Autodesk Fusion 360 part; units mm, degrees
sketch "Sketch1" plane through (0, 0, 0) normal (0, 0, 1) x (1, 0, 0)
  line L0 (9, 9) -> (-9, 9)
  line L1 (-9, 9) -> (-9, -9)
  line L2 (-9, -9) -> (9, -9)
  line L3 (9, -9) -> (9, 9)
  line L4 (9, 9) -> (-9, -9) construction
  line L5 (-9, 9) -> (9, -9) construction
  dimension "d1" = 18
  dimension "d2" = 18
extrude "Extrude1" add sketch "Sketch1" along normal blind 35

Autodesk Fusion 360 part; units mm, degrees
sketch "Sketch1" plane through (0, 0, 0) normal (0, 0, 1) x (1, 0, 0)
  line L0 (-10, -10) -> (10, -10)
  line L1 (10, -10) -> (10, 10)
  line L2 (10, 10) -> (-10, 10)
  line L3 (-10, 10) -> (-10, -10)
  line L4 (-10, -10) -> (10, 10) construction
  line L5 (10, -10) -> (-10, 10) construction
  dimension "d1" = 20
  dimension "d2" = 20
extrude "Extrude1" add sketch "Sketch1" along normal blind 65
sketch "Sketch2" plane through (0, 0, 0) normal (0, 0, -1) x (1, 0, 0)
  line L0 (-10, 10) -> (-10, -10)
  line L1 (-10, -10) -> (10, -10)
  line L2 (10, -10) -> (10, 10)
  line L3 (10, 10) -> (-10, 10)
  line L4 (10, 10) -> (10, -10)
  line L5 (10, -10) -> (10, 10)
  line L6 (10, 10) -> (30, 10) construction
  line L7 (30, 10) -> (30, -10) construction
  line L8 (30, -10) -> (10, -10) construction
  arc A0 (20, -10) -> (20, 10) centre (20, 0) ccw
  line L9 (20, -10) -> (10, -10) construction
  line L10 (10, -10) -> (10, 10) construction
  line L11 (20, -10) -> (10, -10)
  line L12 (20, 10) -> (10, 10)
  point P0 (10, -10)
  point P1 (10, 10)
  dimension "d5" = 20
extrude "Extrude2" add sketch "Sketch2" against normal blind 10 contours L2 L4 L5 A0 L11 L12
sketch "Sketch4" plane through (0, 0, 10) normal (0, 0, 1) x (-1, 0, 0)
  arc A0 (-20, 10) -> (-20, -10) centre (-20, 0) ccw
  line L0 (-20, -10) -> (-10, -10)
  line L1 (-10, -10) -> (-10, 10)
  line L2 (-10, 10) -> (-20, 10)
  line L3 (-20, 10) -> (-20, -10) construction
  point P0 (-20, 10)
  point P1 (-20, -10)
hole "Hole1" at (20, 0, 10) direction (0, 0, -1) diameter 6.5 depth 10 tip angle 180 counterbore diameter 11 counterbore depth 4
sketch "Sketch5" plane through (0, 0, 0) normal (0, 0, -1) x (1, 0, 0)
  circle A0 centre (20, 0) radius 3.25
  line L0 (-10, 10) -> (-10, -10)
  line L1 (-10, -10) -> (20, -10)
  arc A1 (20, -10) -> (20, 10) centre (20, 0) ccw
  line L2 (20, 10) -> (-10, 10)
  line L3 (6, 3.8) -> (-6, 3.8)
  line L4 (-6, 3.8) -> (-6, -3.8)
  line L5 (-6, -3.8) -> (6, -3.8)
  line L6 (6, -3.8) -> (6, 3.8)
  line L7 (6, 3.8) -> (-6, -3.8) construction
  line L8 (-6, 3.8) -> (6, -3.8) construction
  dimension "d13" = 12
  dimension "d14" = 7.6
extrude "Extrude3" add sketch "Sketch5" along normal blind 2 contours L3 L4 L5 L6
fillet "Fillet1" radius 1.5 11 edges at (-10, 10, 32.5) (-10, -10, 32.5) (10, -10, 37.5) (15, -10, 10) (30, 0, 10) (15, 10, 10) (10, 10, 37.5) (6, 3.8, -1) (6, -3.8, -1) (-6, -3.8, -1) (-6, 3.8, -1)
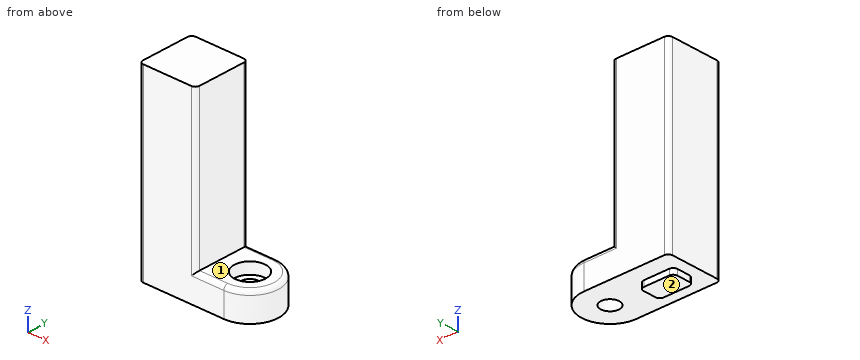
Check sheet for the modelled part. Datum: model origin and axes. Units: mm. Face numbers are marked on the shaded views. A direction names the side the tool comes from. Give positions to 0.01 mm unless a question says otherwise; leave off trailing zeros. Order: outer loops, then holes, each group sorted by start corner. A loop starts at its lowest first (then second) coordinate and runs counter-clockwise, first axis right, second up. Notation, with made-up numbers: M 30.5,3.5 L 87.5,3.5 A23 ccw 87.5,11.5 Z; hole C 30.25,29.5 d3. An arc over 180 degrees is marked long. Answer in a Markdown table with one row per item. Add a question column.
Q1. Sectioned sample at B-B, the plane y = 0. Record the boundary of the cut face in (x, z).
Q2. Gauge pin test, flat ends, axial feed: pin 1 Ø5 at (y, z) = (1.5, 45) entering from +X; pin 2 Ø1 at (y, z) = (6, 8.5) entering from +X; pin 3 Ø5 at (x, y) = (19, -0.5) entering from +Z. Record the tip position at first contact, or that the pin passes through.
Q3. Sectioned sample at A-A, the plane z = 7. Record the boundary of the cut face in (x, y), and give its area (3 significant figures).
Q4. Access from +Z, -Z, +X, -X, +Y, -Y to the whole of each face (thin tool, end or side, straight path). Record for the marked faces 1 and 2.
Q5. Sectioned sample at D-D, the plane x = 1.5. Record the boundary of the cut face in (y, z), and give its area (3 significant figures).
Q6. Sectioned sample at C-C, the plane z = 59. Record the boundary of the cut face in (x, y), and give its area (3 significant figures).
Q7. Thickness scan on L1, parallel to X at y = 0, z = 8.5; L2, parallel to Y at x = 20, z = 7.2; L3, parallel to X at y = 0, z = 1.4. Record the ranges inside material, lowest first.
Verdict:
| question | item | result |
|---|---|---|
| 1 | outline | M -10,0 L -6,0 L -6,-2 L 6,-2 L 6,0 L 16.75,0 L 16.75,6 L 14.5,6 L 14.5,10 L 10,10 L 10,65 L -10,65 Z; M 23.25,0 L 30,0 L 30,8.5 A1.5 ccw 28.5,10 L 25.5,10 L 25.5,6 L 23.25,6 Z |
| 2 | pin 1 | x = 10 |
| 2 | pin 2 | x = 28.35 |
| 2 | pin 3 | z = 6 |
| 3 | outline | M -10,-8.5 A1.5 ccw -8.5,-10 L 20,-10 A10 ccw 20,10 L -8.5,10 A1.5 ccw -10,8.5 Z; hole C 20,0 d11 |
| 3 | area | 661 mm² |
| 4 | face 1 | +Z, +X, +Y, -Y |
| 4 | face 2 | -Z, +X, -X, +Y, -Y |
| 5 | outline | M -10,0 L -3.8,0 L -3.8,-2 L 3.8,-2 L 3.8,0 L 10,0 L 10,65 L -10,65 Z |
| 5 | area | 1,320 mm² |
| 6 | outline | M -10,-8.5 A1.5 ccw -8.5,-10 L 8.5,-10 A1.5 ccw 10,-8.5 L 10,8.5 A1.5 ccw 8.5,10 L -8.5,10 A1.5 ccw -10,8.5 Z |
| 6 | area | 398 mm² |
| 7 | L1 | -10 to 14.5, 25.5 to 30 |
| 7 | L2 | -10 to -5.5, 5.5 to 10 |
| 7 | L3 | -10 to 16.75, 23.25 to 30 |
